Input: part model. Units: mm. Frame: model coordinates. Face numbers are marked on the shaded views. A direction names the side the tool comes from. Give positions to 0.01 mm unless a question says otherwise; leave off trailing zeros. Loops run counter-clockwise (first coordinate to the right, second up) from the corner with the lowest first, then second, coordinate; pieces in that order, holes last. Notation, with made-up numbers: M 35,6 L 52,6 A33 cw 52,34 Z; hole C -11.75,24 d1. An arc over 180 degrees is marked long. Answer as a JSON object with one key per item and string values. Group by question number.
```python
from build123d import *

# Parameters (mm, degrees)
SKETCH1_W                    = 240
SKETCH1_H                    = 2.65684
BASE_FLANGE1_DEPTH           = 60
EDGE_FLANGE1_STRIP_CUT_DEPTH = 240
EDGE_FLANGE1_DEPTH           = 240
EDGE_FLANGE1_START           = 2.65684
EDGE_FLANGE1_FLAT_DEPTH      = 2.65684
CUT_EXTRUDE1_DEPTH           = 33.782
CUT_EXTRUDE1_DEPTH_BACK      = 23.876


# Sheet-metal steps are written as plain solids
with BuildPart() as part:
    # Sketch1 → Base-Flange1 (new body)
    with BuildSketch(Plane.XY):
        with Locations((0, -1.32842)):
            Rectangle(SKETCH1_W, SKETCH1_H)
    extrude(amount=BASE_FLANGE1_DEPTH)

    # Edge-Flange1 strip (across the edge) → Edge-Flange1 strip cut (cut)
    with BuildSketch(Plane(origin=(120, 0, 0), x_dir=(0, 0.7071067811865512, 0.7071067811865438), z_dir=(-1, 0, 0))):
        Polygon((-10.514668246, 6.757329085), (-1.585776362, -2.171562799), (0.292893219, -0.292893219), (-8.635998666, 8.635998666), align=None)
    extrude(amount=EDGE_FLANGE1_STRIP_CUT_DEPTH, mode=Mode.SUBTRACT)

    # Edge-Flange1 bend section (across the edge) → Edge-Flange1 (add)
    with BuildSketch(Plane(origin=(120, 0, 0), x_dir=(0, 0.7071067811865512, 0.7071067811865438), z_dir=(-1, 0, 0))):
        with BuildLine():
            Line((-2.65684, 0.414213562), (0, 0.414213562))
            ThreePointArc((0, 0.414213562), (0.076120467, 0.03153013), (0.292893219, -0.292893219))
            Line((0.292893219, -0.292893219), (-1.585776362, -2.171562799))
            ThreePointArc((-1.585776362, -2.171562799), (-2.37847963, -0.98519852), (-2.65684, 0.414213562))
        make_face()
    extrude(amount=EDGE_FLANGE1_DEPTH)

    # Edge-Flange1 profile (on flange) → Edge-Flange1 flat (add)
    with BuildSketch(Plane(origin=(0, 0, 0), x_dir=(-1, 0, 0), z_dir=(0, -0.7071067811865512, -0.7071067811865438)).offset(EDGE_FLANGE1_START)):
        Polygon((120, 0.414213562), (120, 10), (115.1, 10), (115.1, 13), (110.2, 13), (110.2, 10), (105.3, 10), (105.3, 13), (100.4, 13), (100.4, 10), (95.5, 10), (95.5, 13), (90.6, 13), (90.6, 10), (85.7, 10), (85.7, 13), (80.8, 13), (80.8, 10), (75.9, 10), (75.9, 13), (71, 13), (71, 10), (66.1, 10), (66.1, 13), (61.2, 13), (61.2, 10), (56.3, 10), (56.3, 13), (51.4, 13), (51.4, 10), (46.5, 10), (46.5, 13), (41.6, 13), (41.6, 10), (36.7, 10), (36.7, 13), (31.8, 13), (31.8, 10), (26.9, 10), (26.9, 13), (22, 13), (22, 10), (17.1, 10), (17.1, 13), (12.2, 13), (12.2, 10), (7.3, 10), (7.3, 13), (2.4, 13), (2.4, 10), (-2.5, 10), (-2.5, 13), (-7.4, 13), (-7.4, 10), (-12.3, 10), (-12.3, 13), (-17.2, 13), (-17.2, 10), (-22.1, 10), (-22.1, 13), (-27, 13), (-27, 10), (-31.9, 10), (-31.9, 13), (-36.8, 13), (-36.8, 10), (-41.7, 10), (-41.7, 13), (-46.6, 13), (-46.6, 10), (-51.5, 10), (-51.5, 13), (-56.4, 13), (-56.4, 10), (-61.3, 10), (-61.3, 13), (-66.2, 13), (-66.2, 10), (-71.1, 10), (-71.1, 13), (-76, 13), (-76, 10), (-80.9, 10), (-80.9, 13), (-85.8, 13), (-85.8, 10), (-90.7, 10), (-90.7, 13), (-95.6, 13), (-95.6, 10), (-100.5, 10), (-100.5, 13), (-105.4, 13), (-105.4, 10), (-110.3, 10), (-110.3, 13), (-115.2, 13), (-115.2, 10), (-120, 10), (-120, 0.414213562), align=None)
    extrude(amount=-EDGE_FLANGE1_FLAT_DEPTH)

    # Sketch9 → Cut-Extrude1 (cut, two sides: drawn at the far end of the back side and taken through both)
    with BuildSketch(Plane(origin=(0, 0, 0), x_dir=(1, 0, 0), z_dir=(0, 1, 0)).offset(-CUT_EXTRUDE1_DEPTH_BACK)):
        Polygon((120, -60), (120, 40.593867323), (116.952, 40.593867323), (116.952, -75.248845782), (120, -75.248845782), align=None)
    extrude(amount=CUT_EXTRUDE1_DEPTH + CUT_EXTRUDE1_DEPTH_BACK, mode=Mode.SUBTRACT)


solid = part.part
```
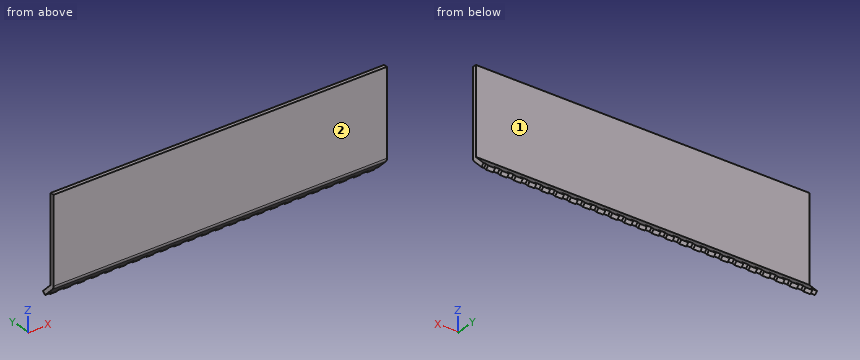
1. Reachability of the marked faces 1 and 2 from +Z, -Z, +X, -X, +Y, -Y: full face, straight path, thin tool, end or side. Return the list, or none.
2. First-contact query: P1, Ø3, axis at y = 8, z = -9.5, coming from the +X side; P2, Ø4, axis at x = 5, y = 3, coming from the +Z side; P3, Ø4, axis at x = 9, y = 6, coming from the -Z side. Flat tips, straight axial feed; report the tip coordinate or a pass-through.
3. Section C-C (y = 2.5). Output: boundary loops of the cut face in (x, z), then the cut area to 3 significant figures.
4. Section B-B (z = 9). Output: boundary loops of the cut face in (x, y), then the cut area to 3 significant figures.
5. Material intervals for L1, parallel to Y at x = 58, z = 27.5; L2, parallel to Y at x = -64, z = -2; L3, parallel to Z at x = 11, y = 1, sorted ascending.
6. Section A-A (x = -53.5). Output: boundary loops of the cut face in (y, z).
Geometry results:
{
 "1": {"face 1": "+Z, +X, -X, +Y", "face 2": "+Z, -Z, +X, -X, -Y"},
 "2": {"P1": "x = 115.2", "P2": "z = -1", "P3": "z = -10.96"},
 "3": {"outline": "M -120,-6.26 L 116.95,-6.26 L 116.95,-2.5 L -120,-2.5 Z", "area": "890 mm2"},
 "4": {"outline": "M -120,-2.66 L 116.95,-2.66 L 116.95,0 L -120,0 Z", "area": "630 mm2"},
 "5": {"L1": "-2.66 to 0", "L2": "-1.75 to 2", "L3": "-4.76 to -1"},
 "6": {"outline": "M -2.66,0.41 A3.66 ccw -1.59,-2.17 L 7.31,-11.07 L 9.19,-9.19 L 0.29,-0.29 A1 cw 0,0.41 L 0,60 L -2.66,60 Z"}
}
